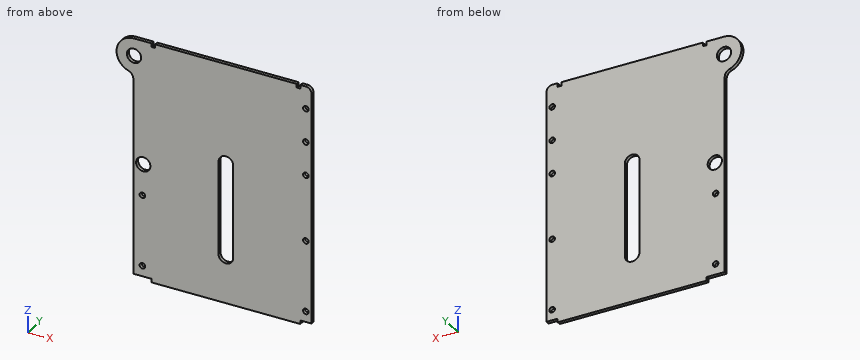
from build123d import *

# Parameters (mm, degrees)
SKETCH002_W     = 266.7
SKETCH002_H     = 430.55
PAD002_DEPTH    = 6.35
SKETCH020_R     = 12.8
SKETCH020_R_2   = 5
PAD014_DEPTH    = 6.35
SKETCH039_W     = 6.75
SKETCH039_H     = 6.55
POCKET_DEPTH    = 6.35
SKETCH056_R     = 5
POCKET002_DEPTH = 100


with BuildPart() as part:
    # Sketch002 (on Face1 of ShapeBinder002) → Pad002 (new body)
    with BuildSketch(Plane.XZ.offset(62.5)):
        with Locations((0, -52.075)):
            Rectangle(SKETCH002_W, SKETCH002_H)
        with BuildLine():
            ThreePointArc((-13.2, -182.35), (0, -195.55), (13.2, -182.35))
            Line((13.2, -182.35), (13.2, -15.975))
            ThreePointArc((13.2, -15.975), (0, -2.775), (-13.2, -15.975))
            Line((-13.2, -15.975), (-13.2, -182.35))
        make_face(mode=Mode.SUBTRACT)
    extrude(amount=PAD002_DEPTH)

    # Sketch020 (on Face10 of Pad002) → Pad014 (join)
    with BuildSketch(Plane.XZ.offset(68.85)):
        with BuildLine():
            Line((-133.35, 163.2), (-149.65, 163.2))
            Line((-164.65, 163.2), (-149.65, 163.2))
            ThreePointArc((-164.65, 163.2), (-195.548892, 136.894842), (-174.511666, 102.19415))
            ThreePointArc((-165.95, 90.330781), (-168.313946, 97.645862), (-174.511666, 102.19415))
            Line((-165.95, -260.9), (-165.95, 90.330781))
            Line((-165.95, -260.9), (-133.35, -260.9))
            Line((-133.35, 163.2), (-133.35, -260.9))
        make_face()
        with Locations((-148.15, -58.775)):
            Circle(SKETCH020_R, mode=Mode.SUBTRACT)
        with Locations((-149.65, -241.95)):
            Circle(SKETCH020_R_2, mode=Mode.SUBTRACT)
        with Locations((-149.65, -114.95)):
            Circle(SKETCH020_R_2, mode=Mode.SUBTRACT)
        with Locations((-164.65, 131.9)):
            Circle(SKETCH020_R, mode=Mode.SUBTRACT)
        with BuildLine():
            Line((133.35, 163.2), (143.35, 163.2))
            ThreePointArc((153.35, 153.2), (150.421068, 160.271068), (143.35, 163.2))
            Line((153.35, 153.2), (153.35, -260.9))
            Line((133.35, -260.9), (153.35, -260.9))
            Line((133.35, -260.9), (133.35, 163.2))
        make_face()
        with Locations((143.35, -241.95)):
            Circle(SKETCH020_R_2, mode=Mode.SUBTRACT)
        with Locations((143.35, -114.95)):
            Circle(SKETCH020_R_2, mode=Mode.SUBTRACT)
    extrude(amount=-PAD014_DEPTH)

    # Sketch039 (on Face22 of Pad014) → Pocket (cut)
    with BuildSketch(Plane.XZ.offset(68.85)):
        with Locations((-130.175, 159.925)):
            Rectangle(SKETCH039_W, SKETCH039_H)
        with Locations((130.175, 159.925)):
            Rectangle(SKETCH039_W, SKETCH039_H)
    extrude(amount=-POCKET_DEPTH, mode=Mode.SUBTRACT)

    # Sketch056 (on Face4 of Pocket) → Pocket002 (cut)
    with BuildSketch(Plane.XZ.offset(68.85)):
        with Locations((143.35, 123.2)):
            Circle(SKETCH056_R)
        with Locations((143.35, 63.2)):
            Circle(SKETCH056_R)
        with Locations((143.35, 3.2)):
            Circle(SKETCH056_R)
    extrude(amount=-POCKET002_DEPTH, mode=Mode.SUBTRACT)


solid = part.part
CAD build for the part. Positions are in the model's coordinates, mm. Give positions to 0.01 mm unless a question says otherwise; leave off trailing zeros. Order: outer loops, then holes, each group sorted by start corner. A loop starts at its lowest first (then second) coordinate and runs counter-clockwise, first axis right, second up. Notation, with made-up numbers: (34, 23.25) -> (57, 23.25) arc R35 ccw to (57, 59.25) -> close; hole circle Ø8 at (10.25, 79.25). An arc over 180 degrees is marked (long way). Return JSON: item names as keys, results as strings.
Q1. Saw through at A-A (z = 63.2). Write the cut outline in (x, y).
Working result:
{"outline": "(-165.95, -68.85) -> (138.35, -68.85) -> (138.35, -62.5) -> (-165.95, -62.5) -> close; (148.35, -68.85) -> (153.35, -68.85) -> (153.35, -62.5) -> (148.35, -62.5) -> close"}
Q2. Flat gauge pins, fed straight in: pin 1 (6 mm diameter, centred on x = -149.65, z = -241.95, fed in from -Y); pin 2 (1.9 mm diameter, centred on y = -65, z = -49, fed in from -X); pin 3 (1.9 mm diameter, centred on y = -66.5, z = -265.5, fed in from +X); pin 4 (3 mm diameter, centred on y = -67, z = 160, fed in from +X). Where does each tip first touch, or does it go through?
Working result:
{"pin 1": "through", "pin 2": "x = -165.95", "pin 3": "x = 133.35", "pin 4": "x = 151.83"}
Q3. Saw through at C-C (z = -241.95). Write the cut outline in (x, y).
Working result:
{"outline": "(-165.95, -68.85) -> (-154.65, -68.85) -> (-154.65, -62.5) -> (-165.95, -62.5) -> close; (-144.65, -68.85) -> (138.35, -68.85) -> (138.35, -62.5) -> (-144.65, -62.5) -> close; (148.35, -68.85) -> (153.35, -68.85) -> (153.35, -62.5) -> (148.35, -62.5) -> close"}
Q4. Saw through at D-D (y = -66.25). Count the separate pieces of the cut face and the enclosed holes in it, then the cut area to 3 significant figures.
Working result:
{"separate pieces": "1", "enclosed holes": "10", "area": "132,000 mm²"}
Q5. Drill centre lines: line 1 (Z direction, x = -149.65, y = -64.25); line 2 (Z direction, x = 143.35, y = -64); line 3 (X direction, y = -65.5, z = -58). Where is each one in solid material? Low to high.
Working result:
{"line 1": "-260.9 to -246.95, -236.95 to -119.95, -109.95 to -71.49, -46.06 to 163.2", "line 2": "-260.9 to -246.95, -236.95 to -119.95, -109.95 to -1.8, 8.2 to 58.2, 68.2 to 118.2, 128.2 to 163.2", "line 3": "-165.95 to -160.93, -135.37 to -13.2, 13.2 to 153.35"}
Q6. Saw through at B-B (x = 0). Write the cut outline in (y, z) (3 decimals).
Working result:
{"outline": "(-68.85, -267.35) -> (-62.5, -267.35) -> (-62.5, -195.55) -> (-68.85, -195.55) -> close; (-68.85, -2.775) -> (-62.5, -2.775) -> (-62.5, 163.2) -> (-68.85, 163.2) -> close"}
